For this review, use the dimensioned drawing (mm, ordinates from the lowest corner) and the shaded views. Give positions to 0.01 mm unless a question says otherwise; leave off trailing zeros. Loops run counter-clockwise (first coordinate to the right, second up) from the corner with the lowest first, then second, coordinate; pieces in that order, holes last. Notation, with made-up numbers: (5.5, 74.25) - (11.5, 74.25) arc R20 ccw to (11.5, 95.25) - close; hole circle Ø10 at (-32.75, 76.25). An arc over 180 degrees is marked (long way). Write each question's results on one line, items separated by ' | '.
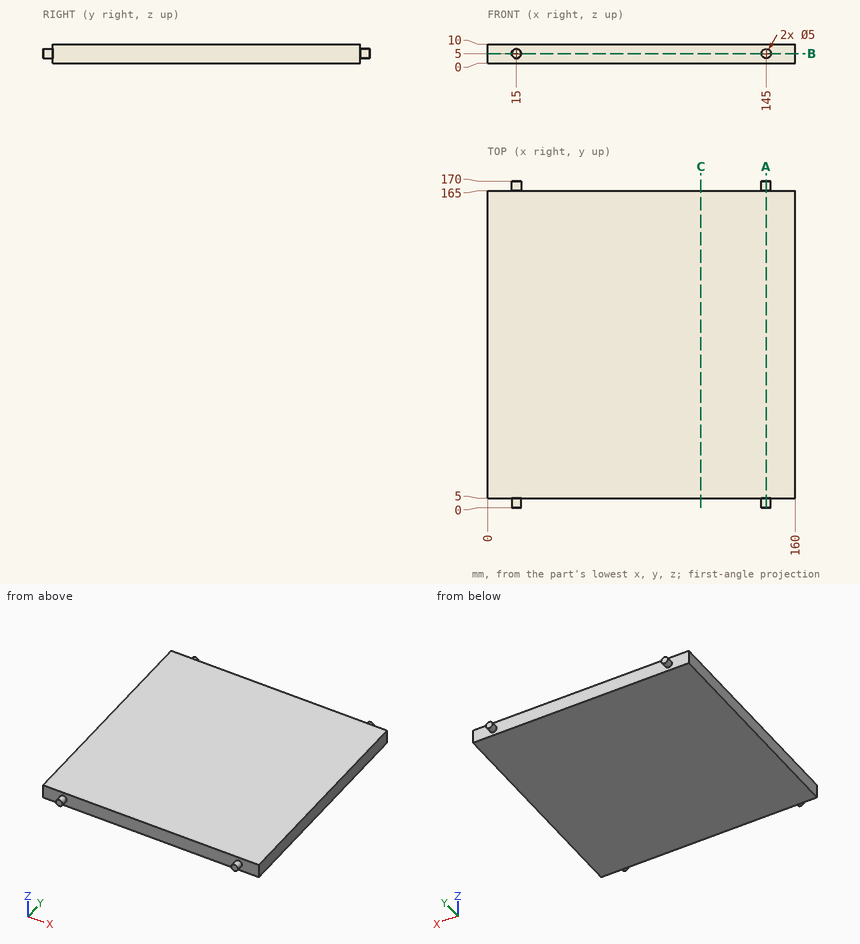
Item 1: Clearance check with flat-ended pins moving along their axes: P1, Ø4, axis at x = 62, z = 4.5, coming from the +Y side; P2, Ø1.5, axis at x = 76, z = 7, coming from the -Y side. State where each tip first meets the part, or that it passes through.
Output values:
P1: stops at y = 165 | P2: stops at y = 5
Item 2: We need section C-C on x = 111. Give the boundary of the cut face in (y, z), then the cut area to 3 significant figures.
Output values:
outline: (5, 0) - (165, 0) - (165, 10) - (5, 10) - close | area: 1,600 mm²
Item 3: We need section B-B on z = 5. Give the boundary of the cut face in (x, y).
Output values:
outline: (0, 5) - (12.5, 5) - (12.5, 0) - (17.5, 0) - (17.5, 5) - (142.5, 5) - (142.5, 0) - (147.5, 0) - (147.5, 5) - (160, 5) - (160, 165) - (147.5, 165) - (147.5, 170) - (142.5, 170) - (142.5, 165) - (17.5, 165) - (17.5, 170) - (12.5, 170) - (12.5, 165) - (0, 165) - close
Item 4: Wall thickness on probe 1 along Y at (x, z) = (86, 3.25): over which ranges is the line inside the solid? List them lowest first.
Output values:
probe 1: y = 5 to 165
Item 5: We need section A-A on x = 145. Give the boundary of the cut face in (y, z), then the cut area to 3 significant figures.
Output values:
outline: (0, 2.5) - (5, 2.5) - (5, 0) - (165, 0) - (165, 2.5) - (170, 2.5) - (170, 7.5) - (165, 7.5) - (165, 10) - (5, 10) - (5, 7.5) - (0, 7.5) - close | area: 1,650 mm²
